Read the model definition and answer for the solid it produces. Units are mm, in the model's axes. Face numbers are marked on the shaded views. A direction names the side the tool comes from. Coordinates: 2 decimals unless noted, no trailing zeros. Write each loop counter-clockwise with the first axis right and the second up, starting at its lowest first coordinate (ties: lowest second). Pieces come first, ordered by that corner, then holes.
1) Find the intervals of material crossed by line 1 (Z direction, x = -7.75, y = -0.5); line 2 (X direction, y = 0, z = 2.5); line 3 (Y direction, x = -2, z = 0), in increasing order.
2) Each of these flat-tipped pins is pushed along its axis until it touches: pin 1 Ø2 at (y, z) = (-1.5, -1.5) entering from -X; pin 2 Ø1 at (y, z) = (3, -0.5) entering from -X; pin 3 Ø4 at (y, z) = (-2.5, -0.5) entering from -X. Where does it stop, or does it pass through?
3) The part is cut by section B-B (y = 0). Determine the outline of the cut face in (x, z).
4) Which of the six approach directions +Z, -Z, +X, -X, +Y, -Y give full straight-line access (tool end or side, diameter ignored) to the marked faces 1 and 2?
5) The part is cut by section D-D (z = -3.25). Determine the outline of the cut face in (x, y).
6) The part is cut by section C-C (x = -9.5). Determine the outline of the cut face in (y, z), then the cut area to 3 significant figures.
7) The part is cut by section A-A (z = 0). Determine the outline of the cut face in (x, y).
8) Determine the mould class of the marked faces 3, 4 and 5 for opening direction X: +X half, -X half, draft (parallel to the pull), parting line (faces both ways), or undercut.
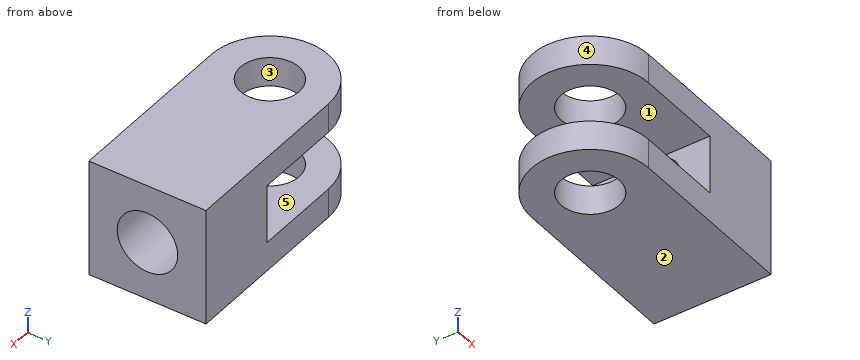
Autodesk Inventor part; units mm, degrees
ref_plane "YZ Plane" through (0, 0, 0) normal (1, 0, 0) x (0, 1, 0)
ref_plane "XZ Plane" through (0, 0, 0) normal (0, 1, 0) x (-1, 0, 0)
ref_plane "XY Plane" through (0, 0, 0) normal (0, 0, 1) x (1, 0, 0)
sketch "Sketch1" plane through (0, 0, 0) normal (0, 0, 1) x (1, 0, 0)
  line L0 (0, 4) -> (-12, 4)
  line L1 (-12, -4) -> (0, -4)
  line L2 (0, -4) -> (0, 4)
  arc A0 (-12, 4) -> (-12, -4) centre (-12, 0) ccw
  point P0 (0, 0)
  point P1 (0, 0)
  dimension "d0" = 4
  dimension "d1" = 12
  dimension "d2" = 8
extrude "Extrusion1" add sketch "Sketch1" along normal mid plane 8
sketch "Sketch3" plane through (0, 0, 4) normal (0, 0, 1) x (1, 0, 0)
  arc A0 (-12, 4) -> (-12, -4) centre (-12, 0) ccw
  point P0 (0, 0)
  point P1 (-12, 0)
hole "Hole1" at (-12, 0, 4) direction (0, 0, -1) diameter 4 depth 8
sketch "Sketch2" plane through (-12, 4, 4) normal (0, 1, 0) x (1, 0, 0)
  line L0 (-4, 6) -> (6, 6)
  line L1 (6, 6) -> (6, 2)
  line L2 (6, 2) -> (-4, 2)
  line L3 (-4, 2) -> (-4, 6)
  line L4 (12, 8) -> (12, 0)
  line L5 (-4, 8) -> (-4, 0)
  point P0 (12, 4)
  point P1 (12, 4)
  point P2 (-4, 4)
  dimension "d5" = 10
  dimension "d6" = 4
extrude "Extrusion2" cut sketch "Sketch2" against normal up to surface (8 mm away)
sketch "Sketch4" plane through (0, -4, 4) normal (1, 0, 0) x (0, 0, -1)
  point P0 (4, 4)
  point P1 (4, 4)
hole "Hole2" at (0, 0, 0) direction (-1, 0, 0) diameter 4.134 depth 6
properties part number "207 part 2"
Reported:
1. line 1: z = -4 to -2, 2 to 4
1. line 2: x = -16 to -14, -10 to 0
1. line 3: y = -4 to -2.07, 2.07 to 4
2. pin 1: stops at x = -15.95
2. pin 2: stops at x = -6
2. pin 3: stops at x = -15.82
3. outline: (-16, -4) - (-14, -4) - (-14, -2) - (-16, -2) - close; (-16, 2) - (-14, 2) - (-14, 4) - (-16, 4) - close; (-10, -4) - (0, -4) - (0, -2.07) - (-6, -2.07) - (-6, -2) - (-10, -2) - close; (-10, 2) - (-6, 2) - (-6, 2.07) - (0, 2.07) - (0, 4) - (-10, 4) - close
4. face 1: -X, +Y, -Y
4. face 2: -Z, +X, -X, +Y, -Y
5. outline: (-12, -4) - (0, -4) - (0, 4) - (-12, 4) arc R4 ccw to start; hole circle Ø4 at (-12, 0)
6. outline: (-4, -4) - (4, -4) - (4, -2) - (-4, -2) - close; (-4, 2) - (4, 2) - (4, 4) - (-4, 4) - close
6. area: 32.0 mm2
7. outline: (-6, -4) - (0, -4) - (0, -2.07) - (-6, -2.07) - close; (-6, 2.07) - (0, 2.07) - (0, 4) - (-6, 4) - close
8. face 3: undercut
8. face 4: -X half
8. face 5: draft
